Verification items for the finished model (mm, model axes). Face numbers are marked on the shaded views. A direction names the side the tool comes from. Give positions to 0.01 mm unless a question says otherwise; leave off trailing zeros. Loops run counter-clockwise (first coordinate to the right, second up) from the corner with the lowest first, then second, coordinate; pieces in that order, holes last. Notation, with made-up numbers: (-14, 55) - (34, 55) arc R25 cw to (34, 72) - close; hole circle Ø3 at (58.25, -33). An arc over 180 degrees is marked (long way). One line per item, written item: value. Start each with the question number.
1. Scan lines: L1, parallel to Z at x = -34.29, y = -15.2; L2, parallel to X at y = 6, z = 45.5 (3 decimals); L3, parallel to Y at x = 18.5, z = 18.5. Record each from-to range of solid material in increasing order. Write a range as [from, to].
2. Sectioned sample at B-B (x = -34.29). Record the cut outline in (y, z).
3. Gauge pin test, flat ends, axial feed: pin 1 (3 mm diameter, centred on x = 33.5, z = 14, fed in from +Y); pin 2 (3.5 mm diameter, centred on x = 24.89, y = 5.02, fed in from +Z); pin 3 (12 mm diameter, centred on y = 12, z = 11, fed in from +X) (3 decimals). Record the tip position at first contact, or that the pin passes through.
4. Sectioned sample at C-C (z = 13). Record the cut outline in (x, y) (1 decimal).
5. Mould release check, pull along Y, two halves, no side actions. Record for the marked faces 4, 5 and 6: pulls with the +Y half, pulls with the -Y half, needs draft (parallel to the pull), parting line crosses it, or undercut.
6. Sectioned sample at D-D (x = 0). Record the cut outline in (y, z).
7. Sectioned sample at A-A (x = -19.5). Record the cut outline in (y, z).
8. Access from +Z, -Z, +X, -X, +Y, -Y to the whole of each face (thin tool, end or side, straight path). Record for the marked faces 1, 2 and 3.
Autodesk Inventor part; units mm, degrees
ref_plane "YZ Plane" through (0, 0, 0) normal (1, 0, 0) x (0, 1, 0)
ref_plane "XZ Plane" through (0, 0, 0) normal (0, 1, 0) x (-1, 0, 0)
ref_plane "XY Plane" through (0, 0, 0) normal (0, 0, 1) x (1, 0, 0)
sketch "Sketch1" plane through (0, 0, 0) normal (0, 0, 1) x (1, 0, 0)
  line L0 (-20.2946, 10.0584) -> (20.2946, 10.0584)
  line L1 (20.2946, 10.0584) -> (20.2946, -10.0584)
  line L2 (20.2946, -10.0584) -> (-20.2946, -10.0584)
  line L3 (-20.2946, -10.0584) -> (-20.2946, 10.0584)
  line L4 (-31.115, 16.8275) -> (31.115, 16.8275)
  line L5 (31.115, 16.8275) -> (31.115, -16.8275)
  line L6 (31.115, -16.8275) -> (-31.115, -16.8275)
  line L7 (-31.115, -16.8275) -> (-31.115, 16.8275)
  circle A0 centre (-24.892, 5.0165) radius 1.5875
  line L8 (0, 0) -> (0, 25.203) construction
  line L9 (0, 0) -> (-28.0291, 0) construction
  circle A1 centre (24.892, 5.0165) radius 1.5875
  line L10 (0, 0) -> (41.5268, 0) construction
  circle A2 centre (-24.892, -5.0165) radius 1.5875
  circle A3 centre (24.892, -5.0165) radius 1.5875
  dimension "d0" = 40.5892
  dimension "d1" = 20.1168
  dimension "d2" = 20.2946
  dimension "d3" = 10.0584
  dimension "d4" = 62.23
  dimension "d5" = 33.655
  dimension "d6" = 16.8275
  dimension "d7" = 31.115
  dimension "d8" = 3.175
  dimension "d9" = 24.892
  dimension "d10" = 5.0165
extrude "Extrusion1" add sketch "Sketch1" along normal blind 1.5875
sketch "Sketch2" plane through (0, 0, 1.5875) normal (0, 0, 1) x (1, 0, 0)
  line L0 (31.115, 16.8275) -> (-31.115, 16.8275)
  line L1 (-31.115, 16.8275) -> (-31.115, -16.8275)
  line L2 (-31.115, -16.8275) -> (31.115, -16.8275)
  line L3 (31.115, -16.8275) -> (31.115, 16.8275)
  line L4 (-28.575, 14.2875) -> (28.575, 14.2875)
  line L5 (28.575, 14.2875) -> (28.575, -14.2875)
  line L6 (28.575, -14.2875) -> (-28.575, -14.2875)
  line L7 (-28.575, -14.2875) -> (-28.575, 14.2875)
  point P0 (0, 0)
  dimension "d13" = 57.15
  dimension "d14" = 28.575
  dimension "d15" = 28.575
  dimension "d16" = 14.2875
extrude "Extrusion2" add sketch "Sketch2" along normal blind 45.466
sketch "Sketch3" plane through (31.115, -16.8275, 0) normal (1, 0, 0) x (0, 0, -1)
  circle A0 centre (-23.114, 25.9715) radius 1.5875
  circle A1 centre (-31.0515, 25.9715) radius 1.5875
  point P0 (0, 16.8275)
  dimension "d19" = 3.175
  dimension "d20" = 9.144
  dimension "d21" = 23.114
  dimension "d22" = 3.175
  dimension "d23" = 9.144
  dimension "d24" = 7.9375
extrude "Extrusion3" cut sketch "Sketch3" against normal through all
sketch "Sketch4" plane through (31.115, -16.8275, 0) normal (1, 0, 0) x (0, 0, -1)
  line L0 (0, 0) -> (0, 33.655)
  line L1 (-47.0535, 0) -> (0, 0)
  line L2 (0, 0) -> (0, 2.54)
  line L3 (0, 2.54) -> (-47.0535, 2.54)
  line L4 (-47.0535, 2.54) -> (-47.0535, 0)
  point P0 (0, 16.8275)
  dimension "d27" = 2.54
extrude "Extrusion4" add sketch "Sketch4" along normal blind 6.35
sketch "Sketch5" plane through (31.115, -14.2875, 47.0535) normal (0, 1, 0) x (1, 0, 0)
  circle A0 centre (3.175, 3.175) radius 1.5875
  line L0 (0, 0) -> (6.35, 0)
  line L1 (6.35, 47.0535) -> (6.35, 0)
  circle A1 centre (3.175, 43.8785) radius 1.5875
  point P0 (-31.115, 47.0535)
  dimension "d30" = 3.175
  dimension "d31" = 3.175
  dimension "d32" = 3.175
  dimension "d33" = 3.175
  dimension "d34" = 3.175
  dimension "d35" = 3.175
extrude "Extrusion5" cut sketch "Sketch5" against normal blind 6.35
sketch "Sketch6" plane through (-31.115, -16.8275, 0) normal (-1, 0, 0) x (0, 0, 1)
  line L0 (0, 0) -> (47.0535, 0)
  line L1 (0, 0) -> (0, 2.54)
  line L2 (0, 0) -> (0, 33.655)
  line L3 (0, 2.54) -> (47.0535, 2.54)
  line L4 (47.0535, 2.54) -> (47.0535, 0)
  point P0 (0, 16.8275)
  dimension "d38" = 2.54
extrude "Extrusion6" add sketch "Sketch6" along normal blind 6.35
sketch "Sketch7" plane through (-31.115, -14.2875, 47.0535) normal (0, 1, 0) x (1, 0, 0)
  circle A0 centre (-3.175, 43.8785) radius 1.5875
  circle A1 centre (-3.175, 3.175) radius 1.5875
  line L0 (-6.35, 0) -> (-6.35, 47.0535)
  point P0 (31.115, 47.0535)
  dimension "d41" = 3.175
  dimension "d42" = 3.175
  dimension "d43" = 3.175
  dimension "d44" = 3.175
  dimension "d45" = 3.175
  dimension "d46" = 3.175
extrude "Extrusion7" cut sketch "Sketch7" against normal blind 6.35
sketch "Sketch8" plane through (-31.115, 16.8275, 0) normal (0, 1, 0) x (1, 0, 0)
  line L0 (62.23, -47.0535) -> (0, -47.0535)
  circle A0 centre (31.115, -43.8785) radius 1.27
  point P0 (31.115, 0)
  dimension "d49" = 2.54
  dimension "d50" = 3.175
  dimension "d51" = 31.115
extrude "Extrusion8" cut sketch "Sketch8" against normal through all
equation "\"d0\" = servL"
equation "\"d1\" = servW"
equation "\"d2\" = 0.5 * servL"
equation "\"d3\" = 0.5 * servW"
equation "\"d4\" = housL + 2 * housT"
equation "\"d5\" = housW + 2 * housT"
equation "\"d6\" = housT + 0.5 * housW"
equation "\"d7\" = housT + 0.5 * housL"
equation "\"d8\" = servMD"
equation "\"d9\" = 0.5 * servML"
equation "\"d10\" = 0.5 * servMW"
equation "\"d11\" = housBT"
equation "\"d13\" = housL"
equation "\"d14\" = housW"
equation "\"d17\" = housH"
equation "\"d19\" = guideD"
equation "\"d22\" = guideD"
equation "\"d24\" = hubH + spoolT"
equation "\"d25\" = housT"
equation "\"d27\" = housT"
equation "\"d38\" = housT"
equation "\"d51\" = 0.5 * housL + housT"
equation "\"spoolD\" = 25.4"
equation "\"hubD\" = 6.35"
equation "\"spoolT\" = 1.5875"
equation "\"hubH\" = 6.35"
equation "\"hornD\" = 25.4"
equation "\"hornT\" = 1.5875"
equation "\"hornS\" = 2.794"
equation "\"hornID\" = 6.096"
equation "\"hornOD\" = 8.89"
equation "\"hornH\" = 2.54"
equation "\"inset\" = 2.032"
equation "\"insetD\" = 5.842"
equation "\"servW\" = 20.1168"
equation "\"servL\" = 40.5892"
equation "\"servML\" = 49.784"
equation "\"servMW\" = 10.033"
equation "\"servMD\" = 3.175"
equation "\"housW\" = 28.575"
equation "\"housL\" = 57.15"
equation "\"housT\" = 2.54"
equation "\"housBT\" = 1.5875"
equation "\"housH\" = 45.466"
equation "\"guideD\" = 3.175"
equation "\"guideH\" = 23.114"
equation "\"guideW\" = 9.144"
properties part number "Housing"
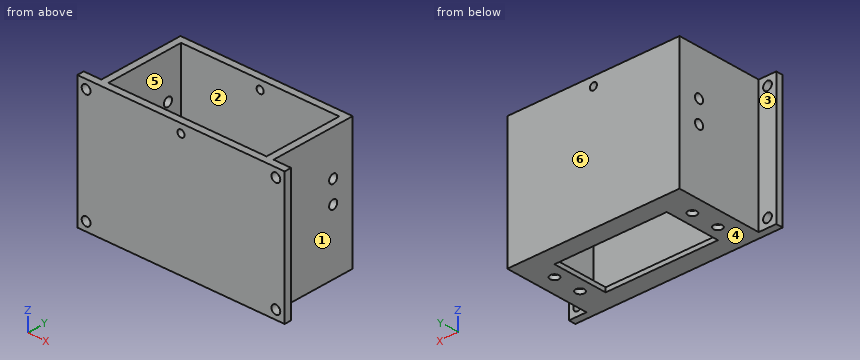
Results are:
1. L1: z = [0, 1.59], [4.76, 42.29], [45.47, 47.05]
1. L2: x = [-31.115, -28.575], [28.575, 31.115]
1. L3: y = [-16.83, -14.29], [14.29, 16.83]
2. outline: (-16.83, 0) - (-14.29, 0) - (-14.29, 1.59) - (-16.83, 1.59) - close; (-16.83, 4.76) - (-14.29, 4.76) - (-14.29, 42.29) - (-16.83, 42.29) - close; (-16.83, 45.47) - (-14.29, 45.47) - (-14.29, 47.05) - (-16.83, 47.05) - close
3. pin 1: stops at y = -14.29
3. pin 2: stops at z = 1.59
3. pin 3: stops at x = 31.115
4. outline: (-37.5, -16.8) - (37.5, -16.8) - (37.5, -14.3) - (31.1, -14.3) - (31.1, 16.8) - (-31.1, 16.8) - (-31.1, -14.3) - (-37.5, -14.3) - close; hole (-28.6, -14.3) - (28.6, -14.3) - (28.6, 14.3) - (-28.6, 14.3) - close
5. face 4: needs draft
5. face 5: undercut
5. face 6: pulls with the +Y half
6. outline: (-16.83, 0) - (-10.06, 0) - (-10.06, 1.59) - (-14.29, 1.59) - (-14.29, 42.61) - (-16.83, 42.61) - close; (-16.83, 45.15) - (-14.29, 45.15) - (-14.29, 47.05) - (-16.83, 47.05) - close; (10.06, 0) - (16.83, 0) - (16.83, 42.61) - (14.29, 42.61) - (14.29, 1.59) - (10.06, 1.59) - close; (14.29, 45.15) - (16.83, 45.15) - (16.83, 47.05) - (14.29, 47.05) - close
7. outline: (-16.83, 0) - (-10.06, 0) - (-10.06, 1.59) - (-14.29, 1.59) - (-14.29, 47.05) - (-16.83, 47.05) - close; (10.06, 0) - (16.83, 0) - (16.83, 47.05) - (14.29, 47.05) - (14.29, 1.59) - (10.06, 1.59) - close
8. face 1: +Z, -Z, +X, +Y
8. face 2: +Z
8. face 3: +Z, -Z, -X, +Y
